Here's the drawing with two shaded views (mm, measured from the low corner). I have some questions. A direction names the side the tool comes from. Coordinates: 2 decimals unless noted, no trailing zeros. Order: outer loops, then holes, each group sorted by start corner. A loop starts at its lowest first (then second) coordinate and runs counter-clockwise, first axis right, second up. Notation, with made-up numbers: (-27, 24) - (24, 24) arc R29 ccw to (24, 51) - close; hole circle Ø7 at (23.25, 77.25). An arc over 180 degrees is marked (long way). Answer as a JSON object with one key per item and string values. Group by question number.
(1) Will these pins go through, and if not, where does the flat tip stop? P1, Ø6, axis at x = 32, y = 28, coming from the -Z side; P2, Ø2, axis at x = 18.5, z = 3, coming from the -Y side; P3, Ø1, axis at y = 29, z = 3, coming from the +X side.
(2) Which directions (+Z, -Z, +X, -X, +Y, -Y) give clear straight access to the entire face, cutting with the end or side of a thin tool? Please do the marked faces 5 and 6.
(3) Imagine slicing it at A-A, the plane z = 1.5. Write out the boundary of the cut face in (x, y), and give its area (3 significant figures).
(4) Imagine slicing it at D-D, the plane y = 8.5. Write out the boundary of the cut face in (x, z).
(5) Please list where these lines run through material, in increasing order: probe 1 along X at (y, z) = (6, 0.5); probe 2 along X at (y, z) = (32, 4.75) (1 decimal); probe 3 along Y at (x, z) = (24, 4.25).
(6) Imagine slicing it at B-B, the plane x = 25. Write out the boundary of the cut face in (y, z).
(7) We'd pull the mould along Y, two halves only. Please class the marked faces 1, 2, 3 and 4: pulls with the +Y half, pulls with the -Y half, needs draft (parallel to the pull), parting line crosses it, or undercut.
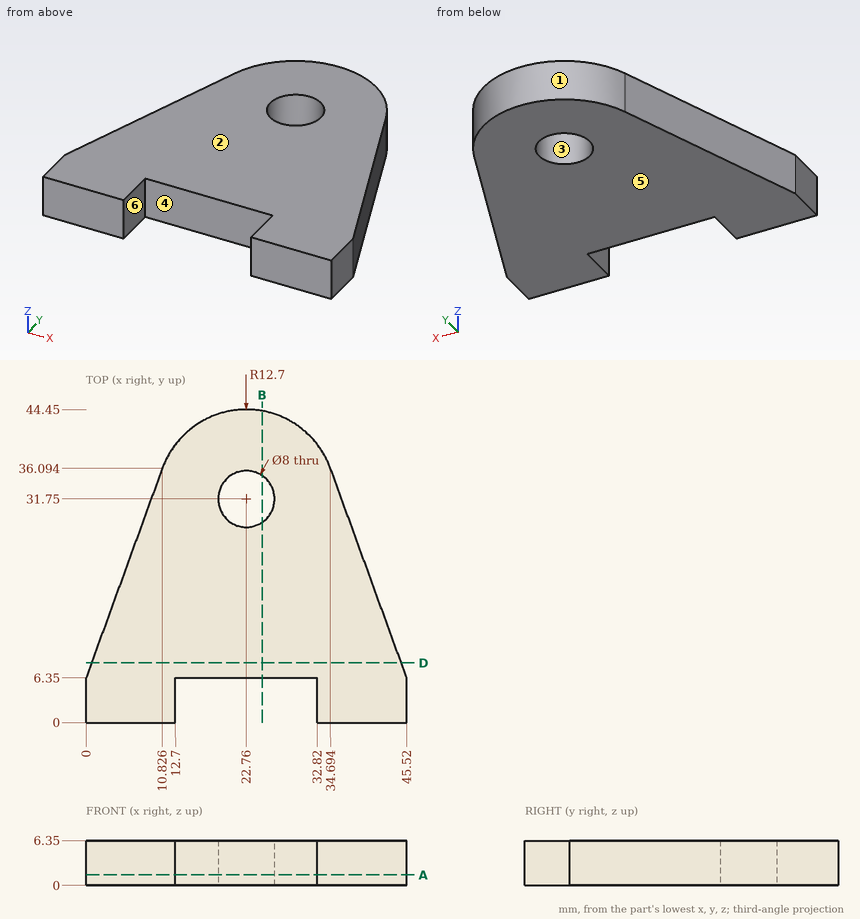
Result set:
{
 "1": {"P1": "stops at z = 0", "P2": "stops at y = 6.35", "P3": "stops at x = 37.46"},
 "2": {"face 5": "-Z, +X, -X, +Y, -Y", "face 6": "+Z, -Z, -Y"},
 "3": {"outline": "(0, 0) - (12.7, 0) - (12.7, 6.35) - (32.82, 6.35) - (32.82, 0) - (45.52, 0) - (45.52, 6.35) - (34.69, 36.09) arc R12.7 ccw to (10.83, 36.09) - (0, 6.35) - close; hole circle Ø8 at (22.76, 31.75)", "area": "1,290 mm^2"},
 "4": {"outline": "(0.78, 0) - (44.74, 0) - (44.74, 6.35) - (0.78, 6.35) - close"},
 "5": {"probe 1": "x = 0 to 12.7, 32.82 to 45.52", "probe 2": "x = 9.3 to 18.8, 26.8 to 36.2", "probe 3": "y = 6.35 to 27.95, 35.55 to 44.39"},
 "6": {"outline": "(6.35, 0) - (28.44, 0) - (28.44, 6.35) - (6.35, 6.35) - close; (35.06, 0) - (44.25, 0) - (44.25, 6.35) - (35.06, 6.35) - close"},
 "7": {"face 1": "pulls with the +Y half", "face 2": "needs draft", "face 3": "undercut", "face 4": "pulls with the -Y half"}
}
